Input: part model. Units: mm. Frame: model coordinates. A direction names the side the tool comes from. Coordinates: 2 decimals unless noted, no trailing zeros. Order: outer loops, then holes, each group sorted by start corner. A loop starts at its lowest first (then second) coordinate and runs counter-clockwise, first axis right, second up.
from build123d import *

# Parameters (mm, degrees)
F1_DEPTH = 5
F3_DEPTH = 3
F4_R     = 3


with BuildPart() as f1:
    # F0 (on Top) → F1 (new body)
    with BuildSketch(Plane.XY):
        Polygon((-44, 11.5), (-44, 0), (-44, -11.5), (0, -11.5), (44, -11.5), (44, 0), (44, 11.5), (0, 11.5), align=None)
        Polygon((-20, 5.5), (-20, 0), (-20, -5.5), (-38, -5.5), (-38, 0), (-38, 5.5), align=None, mode=Mode.SUBTRACT)
        Polygon((20, -5.5), (20, 0), (20, 5.5), (38, 5.5), (38, 0), (38, -5.5), align=None, mode=Mode.SUBTRACT)
    extrude(amount=F1_DEPTH)

    # F2 (on face) → F3 (join)
    with BuildSketch(Plane.XY.offset(5)):
        Polygon((-44, 11.5), (-44, 0), (-44, -11.5), (-14, -11.5), (-14, 0), (-14, 11.5), align=None)
        Polygon((-41, 5.5), (-38, 5.5), (-20, 5.5), (-17, 5.5), (-17, 0), (-17, -5.5), (-20, -5.5), (-38, -5.5), (-41, -5.5), (-41, 0), align=None, mode=Mode.SUBTRACT)
        Polygon((14, 11.5), (-14, 11.5), (-14, 0), (-14, -11.5), (14, -11.5), (14, 0), align=None)
        Polygon((44, 11.5), (14, 11.5), (14, 0), (14, -11.5), (44, -11.5), (44, 0), align=None)
        Polygon((17, 0), (17, 5.5), (41, 5.5), (41, 0), (41, -5.5), (17, -5.5), align=None, mode=Mode.SUBTRACT)
    extrude(amount=F3_DEPTH)

    # F4
    f4_edges = [f1.edges().sort_by_distance(p)[0] for p in [
        (0, -11.5, 0),
        (0, 11.5, 0),
    ]]
    fillet(f4_edges, radius=F4_R)


solid = f1.part
Item 1: Cut plane B-B on y = 1.75. Return loops of the section in (x, z), then the cut area to 3 significant figures.
Response values:
outline: (-44, 0) - (-38, 0) - (-38, 5) - (-41, 5) - (-41, 8) - (-44, 8) - close; (-20, 0) - (20, 0) - (20, 5) - (17, 5) - (17, 8) - (-17, 8) - (-17, 5) - (-20, 5) - close; (38, 0) - (44, 0) - (44, 8) - (41, 8) - (41, 5) - (38, 5) - close
area: 380 mm2
Item 2: Pin query (flat end, axial travel): pin 1 Ø1.5 at (x, y) = (-39.5, 0.5) entering from +Z; pin 2 Ø1 at (x, z) = (0, 2) entering from -Y. Return the tip coordinate at first contact, or that it passes through.
Response values:
pin 1: stops at z = 5
pin 2: stops at y = -11.46
Item 3: Draft query along Y for faces 1 (the face through (-29, 5.5, 4)), 2 (the face through (44, 0, 4)), 3 (the face through (-41, 0, 6)), 4 (the face through (-1, -11.5, 5)). Return one class per face: pulls with the +Y half, pulls with the -Y half, needs draft (parallel to the pull), parting line crosses it, or undercut.
Response values:
face 1: undercut
face 2: needs draft
face 3: undercut
face 4: pulls with the -Y half
Item 4: Cut plane D-D on x = -12. Return loops of the section in (y, z), then the cut area to 3 significant figures.
Response values:
outline: (-11.5, 3) arc R3 ccw to (-8.5, 0) - (8.5, 0) arc R3 ccw to (11.5, 3) - (11.5, 8) - (-11.5, 8) - close
area: 180 mm2
Item 5: Access query for faces 5 (the face through (-20, 0, 2)), 6 (the face through (18, 0, 5)), 7 (the face through (-0.62, 10.6, 0.86)). Directions: +Z, -Z, +X, -X, +Y, -Y. A direction counts if a zero-diameter tool reaches every point of the face in a straight line with its end or side. Return the directions, or none.
Response values:
face 5: +Z, -Z
face 6: +Z
face 7: -Z, +X, -X, +Y
Item 6: Cut plane A-A on x = -24. Return loops of the section in (y, z).
Response values:
outline: (-11.5, 3) arc R3 ccw to (-8.5, 0) - (-5.5, 0) - (-5.5, 8) - (-11.5, 8) - close; (5.5, 0) - (8.5, 0) arc R3 ccw to (11.5, 3) - (11.5, 8) - (5.5, 8) - close
Item 7: Ray query, probe 1 along X at (y, z) = (-1.25, 3); probe 2 along X at (y, z) = (4.75, 6.75); probe 3 along Y at (x, z) = (39, 6.25). Return the intervals inside material, ascending.
Response values:
probe 1: x = -44 to -38, -20 to 20, 38 to 44
probe 2: x = -44 to -41, -17 to 17, 41 to 44
probe 3: y = -11.5 to -5.5, 5.5 to 11.5
Item 8: Cut plane C-C on z = 6.75. Return loops of the section in (x, y).
Response values:
outline: (-44, -11.5) - (44, -11.5) - (44, 11.5) - (-44, 11.5) - close; hole (-41, -5.5) - (-17, -5.5) - (-17, 5.5) - (-41, 5.5) - close; hole (17, -5.5) - (41, -5.5) - (41, 5.5) - (17, 5.5) - close
